Part model, mm, in its own coordinate system. Face numbers are marked on the shaded views. Coordinates: 2 decimals unless noted, no trailing zeros. Write each loop counter-clockwise with the first axis right and the second up, starting at its lowest first coordinate (ties: lowest second). Pieces come first, ordered by that corner, then holes. Notation, with made-up numbers: M -38,-40 L -2,-40 A30 cw -2,-10 Z; hole C -16.5,9.25 d6. An arc over 180 degrees is marked long. Use a Markdown table: item, result. Add a question column.
Q1. Slice it at B-B on z = -180.5. Write the cut outline in (x, y), then the cut area to 3 significant figures.
Q2. Slice it at A-A on y = 163. Write the cut outline in (x, z), then the cut area to 3 significant figures.
Q3. Slice it at C-C on x = 188.5. Write the cut outline in (y, z), then the cut area to 3 significant figures.
Q4. Slice it at D-D on y = 21. Write the cut outline in (x, z), then the cut area to 3 significant figures.
Q5. Pin check, flat tips, straight feed: pin 1 Ø5.5 at (x, z) = (43.5, 117.66) entering from -Y; pin 2 Ø5 at (x, y) = (21.86, 30) entering from -Z; pin 3 Ø5 at (x, y) = (-88, 29.5) entering from +Z; pin 4 Ø5 at (y, z) = (75, 66.25) entering from +X. Stop position of each tip, or through.
Q6. Wall check: L1, parallel to X at y = 156.5, z = 48; L2, parallel to Z at x = -31.5, y = 30; L3, parallel to Y at x = -31, z = -196.5. Give the ranges that are in metal, low to high. Write a range as from..to.
Q7. Mould opens along Z. For the marked faces 1 and 2 say: released by +Z, released by -Z, zero draft, split by the parting line, or undercut.
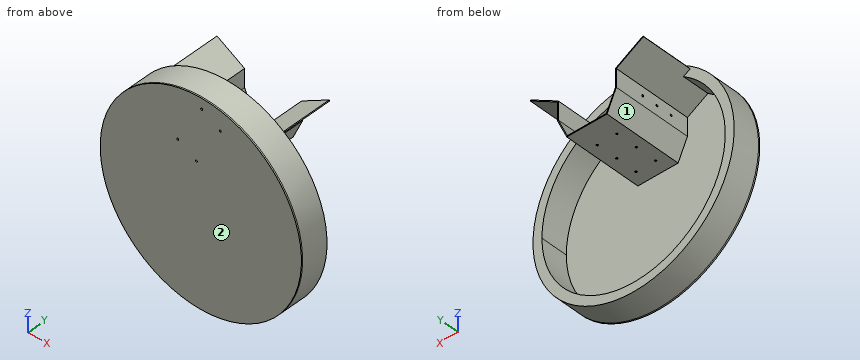
from build123d import *

# Parameters (mm, degrees)
EXTRUDE_THIN1_DEPTH = 175
CUT_EXTRUDE1_REACH  = 249.104
SKETCH2_R           = 2.1
CUT_EXTRUDE2_REACH  = 224.775
SKETCH3_R           = 2.25
SKETCH4_R           = 225
BOSS_EXTRUDE1_DEPTH = 3
SKETCH5_R           = 2.2
CUT_EXTRUDE3_DEPTH  = 3
BOSS_EXTRUDE2_START = 60
SKETCH6_R           = 225
SKETCH6_R_2         = 205
BOSS_EXTRUDE2_DEPTH = 60


with BuildPart() as part:
    # Sketch1 → Extrude-Thin1 (new body)
    with BuildSketch(Plane(origin=(0, 0, 0), x_dir=(1, 0, 0), z_dir=(0, 1, 0))):
        Polygon((0, 0), (-45, 0), (-65.833333333, -45.452967144), (-65.833333333, -85.452967144), (-126.455111598, -120.452967144), (-125.455111598, -122.185017952), (-63.833333333, -86.607667683), (-63.833333333, -45.889482298), (-43.716622104, -2), (0, -2), align=None)
    extrude_thin1 = extrude(amount=EXTRUDE_THIN1_DEPTH)

    # Sketch2 → Cut-Extrude1 (cut, up to next)
    with BuildSketch(Plane.XY.offset(2), mode=Mode.PRIVATE) as cut_extrude1_sk1:
        with Locations((-21.858311052, 30)):
            Circle(SKETCH2_R)
    cut_extrude1_tool1 = extrude(cut_extrude1_sk1.sketch, amount=-CUT_EXTRUDE1_REACH, mode=Mode.PRIVATE) & part.part
    # Sketch2 → Cut-Extrude1 (cut, up to next)
    with BuildSketch(Plane.XY.offset(2), mode=Mode.PRIVATE) as cut_extrude1_sk2:
        with Locations((-21.858311052, 77.5)):
            Circle(SKETCH2_R)
    cut_extrude1_tool2 = extrude(cut_extrude1_sk2.sketch, amount=-CUT_EXTRUDE1_REACH, mode=Mode.PRIVATE) & part.part
    # Sketch2 → Cut-Extrude1 (cut, up to next)
    with BuildSketch(Plane.XY.offset(2), mode=Mode.PRIVATE) as cut_extrude1_sk3:
        with Locations((-21.858311052, 125)):
            Circle(SKETCH2_R)
    cut_extrude1_tool3 = extrude(cut_extrude1_sk3.sketch, amount=-CUT_EXTRUDE1_REACH, mode=Mode.PRIVATE) & part.part
    cut_extrude1_1 = cut_extrude1_tool1.solids().sort_by_distance((-21.858311, 30, 2))[0]
    add(cut_extrude1_1, mode=Mode.SUBTRACT)
    cut_extrude1_2 = cut_extrude1_tool2.solids().sort_by_distance((-21.858311, 77.5, 2))[0]
    add(cut_extrude1_2, mode=Mode.SUBTRACT)
    cut_extrude1_3 = cut_extrude1_tool3.solids().sort_by_distance((-21.858311, 125, 2))[0]
    add(cut_extrude1_3, mode=Mode.SUBTRACT)
    cut_extrude1 = cut_extrude1_1 + cut_extrude1_2 + cut_extrude1_3  # Cut-Extrude1 as one shape, for the pattern or mirror that repeats it

    # Sketch3 → Cut-Extrude2 (cut, up to next)
    with BuildSketch(Plane(origin=(-63.833333333, 0, 0), x_dir=(0, 0, -1), z_dir=(1, 0, 0)), mode=Mode.PRIVATE) as cut_extrude2_sk1:
        with Locations((-66.248574991, 40)):
            Circle(SKETCH3_R)
    cut_extrude2_tool1 = extrude(cut_extrude2_sk1.sketch, amount=-CUT_EXTRUDE2_REACH, mode=Mode.PRIVATE) & part.part
    # Sketch3 → Cut-Extrude2 (cut, up to next)
    with BuildSketch(Plane(origin=(-63.833333333, 0, 0), x_dir=(0, 0, -1), z_dir=(1, 0, 0)), mode=Mode.PRIVATE) as cut_extrude2_sk2:
        with Locations((-66.248574991, 75)):
            Circle(SKETCH3_R)
    cut_extrude2_tool2 = extrude(cut_extrude2_sk2.sketch, amount=-CUT_EXTRUDE2_REACH, mode=Mode.PRIVATE) & part.part
    # Sketch3 → Cut-Extrude2 (cut, up to next)
    with BuildSketch(Plane(origin=(-63.833333333, 0, 0), x_dir=(0, 0, -1), z_dir=(1, 0, 0)), mode=Mode.PRIVATE) as cut_extrude2_sk3:
        with Locations((-66.248574991, 110)):
            Circle(SKETCH3_R)
    cut_extrude2_tool3 = extrude(cut_extrude2_sk3.sketch, amount=-CUT_EXTRUDE2_REACH, mode=Mode.PRIVATE) & part.part
    cut_extrude2_1 = cut_extrude2_tool1.solids().sort_by_distance((-63.833333, 40, 66.248575))[0]
    add(cut_extrude2_1, mode=Mode.SUBTRACT)
    cut_extrude2_2 = cut_extrude2_tool2.solids().sort_by_distance((-63.833333, 75, 66.248575))[0]
    add(cut_extrude2_2, mode=Mode.SUBTRACT)
    cut_extrude2_3 = cut_extrude2_tool3.solids().sort_by_distance((-63.833333, 110, 66.248575))[0]
    add(cut_extrude2_3, mode=Mode.SUBTRACT)
    cut_extrude2 = cut_extrude2_1 + cut_extrude2_2 + cut_extrude2_3  # Cut-Extrude2 as one shape, for the pattern or mirror that repeats it

    # Mirror1: Extrude-Thin1, Cut-Extrude1, Cut-Extrude2 across plane
    add(extrude_thin1.mirror(Plane(origin=(0, 0, 0), x_dir=(0, 0, 1), z_dir=(1, 0, 0))))
    add(cut_extrude1.mirror(Plane(origin=(0, 0, 0), x_dir=(0, 0, 1), z_dir=(1, 0, 0))), mode=Mode.SUBTRACT)
    add(cut_extrude2.mirror(Plane(origin=(0, 0, 0), x_dir=(0, 0, 1), z_dir=(1, 0, 0))), mode=Mode.SUBTRACT)

    # Sketch4 → Boss-Extrude1 (add)
    with BuildSketch(Plane.XZ):
        with Locations(Location((0, -60, 0), (0, 0, 270))):
            Circle(SKETCH4_R)
    extrude(amount=BOSS_EXTRUDE1_DEPTH)

    # Sketch5 → Cut-Extrude3 (cut)
    with BuildSketch(Plane(origin=(0, 0, 0), x_dir=(1, 0, 0), z_dir=(0, 1, 0))):
        with Locations(Location((-10, -25, 0), (0, 0, 270))):
            Circle(SKETCH5_R)
        with Locations(Location((43.5, -117.664718205, 0), (0, 0, 270))):
            Circle(SKETCH5_R)
        with Locations(Location((1.930780618, -141.664718205, 0), (0, 0, 270))):
            Circle(SKETCH5_R)
        with Locations(Location((-51.569219382, -49, 0), (0, 0, 270))):
            Circle(SKETCH5_R)
    extrude(amount=-CUT_EXTRUDE3_DEPTH, mode=Mode.SUBTRACT)

    # Sketch6 → Boss-Extrude2 (add)
    with BuildSketch(Plane(origin=(0, 0, 0), x_dir=(1, 0, 0), z_dir=(0, 1, 0)).offset(BOSS_EXTRUDE2_START)):
        with Locations(Location((0, 60, 0), (0, 0, 270))):
            Circle(SKETCH6_R)
        with Locations((0, 60)):
            Circle(SKETCH6_R_2, mode=Mode.SUBTRACT)
    extrude(amount=-BOSS_EXTRUDE2_DEPTH)


solid = part.part
Recorded:
| question | item | result |
|---|---|---|
| 1 | outline | M -190.01,-3 L 190.01,-3 L 190.01,60 L 165.85,60 L 165.85,0 L -165.85,0 L -165.85,60 L -190.01,60 Z |
| 1 | area | 4,040 mm² |
| 2 | outline | M -126.46,120.45 L -65.83,85.45 L -65.83,45.45 L -45,0 L 45,0 L 65.83,45.45 L 65.83,85.45 L 126.46,120.45 L 125.46,122.19 L 63.83,86.61 L 63.83,45.89 L 43.72,2 L -43.72,2 L -63.83,45.89 L -63.83,86.61 L -125.46,122.19 Z |
| 2 | area | 818 mm² |
| 3 | outline | M -3,-182.85 L 60,-182.85 L 60,-140.58 L 0,-140.58 L 0,20.58 L 60,20.58 L 60,62.85 L -3,62.85 Z |
| 3 | area | 5,810 mm² |
| 4 | outline | C 0,-60 d450; hole M -111.67,111.92 A205 ccw long 111.67,111.92 L 65.83,85.45 L 65.83,45.45 L 45,0 L -45,0 L -65.83,45.45 L -65.83,85.45 Z; hole M -109.77,113.13 L -63.83,86.61 L -63.83,45.89 L -43.72,2 L 43.72,2 L 63.83,45.89 L 63.83,86.61 L 109.77,113.13 A205 ccw Z |
| 4 | area | 27,800 mm² |
| 5 | pin 1 | y = -3 |
| 5 | pin 2 | z = -284.17 |
| 5 | pin 3 | z = 148.12 |
| 5 | pin 4 | x = 65.83 |
| 6 | L1 | -65.83..-63.83, 63.83..65.83 |
| 6 | L2 | -282.78..-262.57, 0..2, 142.57..162.78 |
| 6 | L3 | -3..0 |
| 7 | face 1 | undercut |
| 7 | face 2 | zero draft |
